Model file for the job. Use its own axes, mm. A direction names the side the tool comes from. Round coordinates to 2 decimals unless told otherwise and drop trailing zeros. Order: outer loops, then holes, each group sorted by start corner. A loop starts at its lowest first (then second) coordinate and runs counter-clockwise, first axis right, second up. Notation, with made-up numbers: (23, 65.5) -> (73, 65.5) arc R17 cw to (73, 80.5) -> close; hole circle Ø6 at (11.5, -5). An arc over 180 degrees is marked (long way). Answer as CSV lines item,"result".
Autodesk Inventor part; units mm, degrees
ref_plane "YZ Plane" through (0, 0, 0) normal (1, 0, 0) x (0, 1, 0)
ref_plane "XZ Plane" through (0, 0, 0) normal (0, 1, 0) x (-1, 0, 0)
ref_plane "XY Plane" through (0, 0, 0) normal (0, 0, 1) x (1, 0, 0)
sketch "Sketch1" plane through (0, 0, 0) normal (0, 0, 1) x (1, 0, 0)
  line L0 (0, 0) -> (6.2, 0)
  line L1 (6.2, 0) -> (6.2, 6.2)
  line L2 (6.2, 6.2) -> (0, 6.2)
  line L3 (0, 6.2) -> (0, 0)
  line L4 (0, 6.2) -> (6.2, 0) construction
  line L5 (6.2, 6.2) -> (0, 0) construction
  circle A0 centre (3.1, 3.1) radius 1.75
  dimension "d0" = 6.2
  dimension "d1" = 6.2
  dimension "d2" = 3.5
extrude "Extrusion1" add sketch "Sketch1" along normal blind 3.5 contours L3 L2 L1 L0 | A0
extrude "Extrusion2" add sketch "Sketch1" against normal blind 1.5 contours A0
fillet "Fillet1" radius 0.4 4 edges at (0, 6.2, 1.75) (0, 0, 1.75) (6.2, 0, 1.75) (6.2, 6.2, 1.75)
fillet "Fillet2" radius 0.25 1 edges at (1.35, 3.1, -1.5)
properties part number "Button"
Q1. Saw through at C-C (z = -0.65). Write the cut outline in (x, y).
Checks:
outline,"circle Ø3.5 at (3.1, 3.1)"
Q2. Saw through at A-A (y = 3.1). Write the cut outline in (x, z), plus the area to 3 significant figures.
Checks:
outline,"(0, 0) -> (1.35, 0) -> (1.35, -1.25) arc R0.25 ccw to (1.6, -1.5) -> (4.6, -1.5) arc R0.25 ccw to (4.85, -1.25) -> (4.85, 0) -> (6.2, 0) -> (6.2, 3.5) -> (0, 3.5) -> close"
area,"26.9 mm²"
Q3. Saw through at D-D (x = 5.5). Write the cut outline in (y, z).
Checks:
outline,"(0, 0) -> (6.2, 0) -> (6.2, 3.5) -> (0, 3.5) -> close"
Q4. Wall check: L1, parallel to Z at x = 2.75, y = 5.5; L2, parallel to Y at x = 2.75, z = -1.1; L3, parallel to X at y = 3.5, z = -0.35. Give the ranges that are in metal, low to high. Write a range as [from, to].
Checks:
L1,"[0, 3.5]"
L2,"[1.39, 4.81]"
L3,"[1.4, 4.8]"
Q5. Tool access for faces 1 (the flat face through (0, 3, 2)), 2 (the cylindrical face through (1.35, 3.18, -0.62)): list every direction of +Z, -Z, +X, -X, +Y, -Y with a clear straight run to the whole face (end or side of a thin tool).
Checks:
face 1,"+Z, -Z, -X, +Y, -Y"
face 2,"-Z"
Q6. Flat gauge pins, fed straight in: pin 1 (2 mm diameter, centred on x = 5.5, y = 4, fed in from -Z); pin 2 (1 mm diameter, centred on y = 2.5, z = -1, fed in from -X). Where does each tip first touch, or does it go through?
Checks:
pin 1,"z = -1.49"
pin 2,"x = 1.35"
